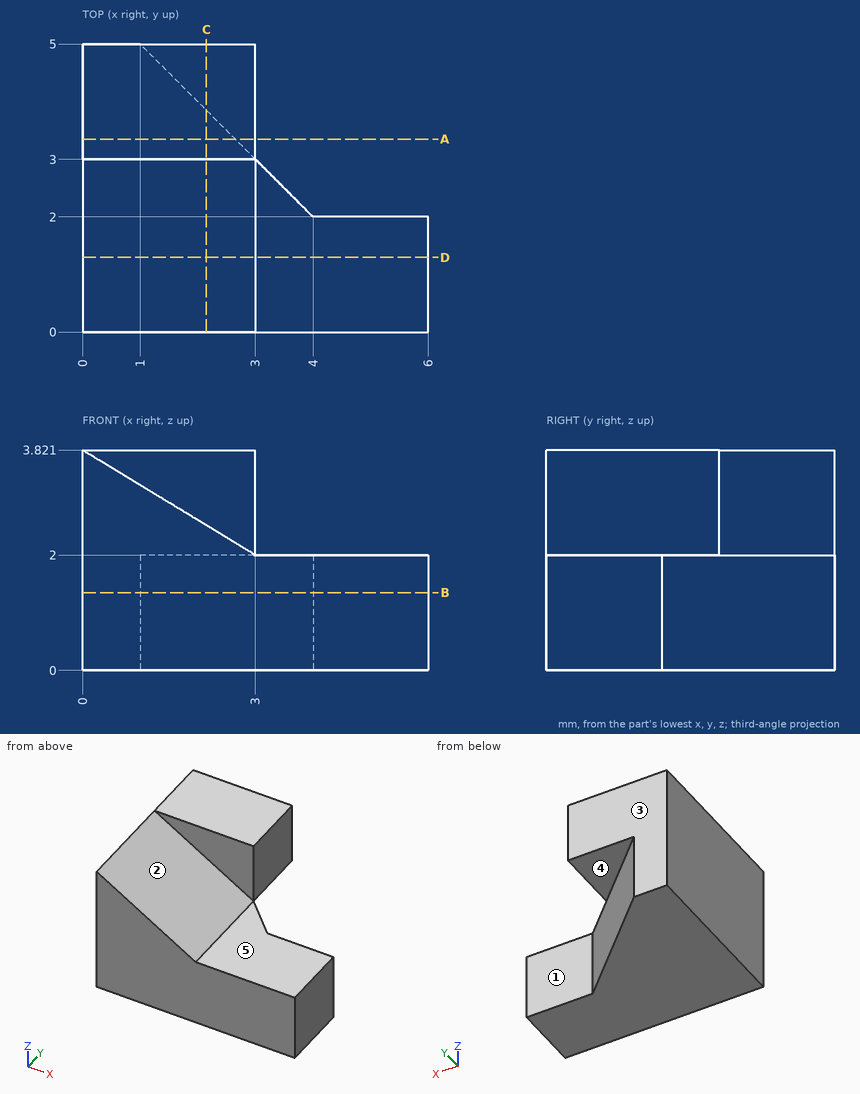
Geometry check sheet. Reference: drawing and pictorial views, mm from the part's lowest x, y, z. A direction names the side the tool comes from. Round coordinates to 2 decimals unless told otherwise and drop trailing zeros. Loops run counter-clockwise (first coordinate to the right, second up) from the corner with the lowest first, then second, coordinate; pieces in that order, holes last. Notation, with made-up numbers: (39.5, 4.5) -> (64.5, 4.5) arc R6 cw to (64.5, 9.5) -> close; hole circle Ø2 at (70.25, -3). An arc over 180 degrees is marked (long way). Use a Markdown table: item, result.
(1) Set-up check for the marked faces 1, 2, 3, 4 and 5: record each of +Z, -Z, +X, -X, +Y, -Y from which the full face is reachable in a straight line by a thin tool's end or side.
Calculated:
| item | result |
|---|---|
| face 1 | +Z, -Z, +X, +Y |
| face 2 | +Z, +X, -Y |
| face 3 | +Z, -Z, +X, -X, +Y |
| face 4 | -Z, +X, +Y |
| face 5 | +Z, +X, +Y, -Y |
(2) Go/stop test with flat-tipped pins: P1, Ø2, axis at y = 4, z = 0.5, coming from the +X side; P2, Ø1.5, axis at x = 5, y = 1.5, coming from the +Z side; P3, Ø2, axis at x = 5, z = 2.5, coming from the +Y side. Record where each tip stops, or that it passes through.
Calculated:
| item | result |
|---|---|
| P1 | x = 3 |
| P2 | z = 2 |
| P3 | y = 2 |
(3) Sectioned sample at B-B (z = 1.35). Enter the section's corners in (x, y).
Calculated:
| item | result |
|---|---|
| outline | (0, 0) -> (6, 0) -> (6, 2) -> (4, 2) -> (1, 5) -> (0, 5) -> close |
(4) Sectioned sample at A-A (y = 3.35). Enter the section's corners in (x, z), then the cut area to 3 significant figures.
Calculated:
| item | result |
|---|---|
| outline | (0, 0) -> (2.65, 0) -> (2.65, 2) -> (3, 2) -> (3, 3.82) -> (0, 3.82) -> close |
| area | 10.8 mm² |
(5) Sectioned sample at D-D (y = 1.3). Enter the section's corners in (x, z).
Calculated:
| item | result |
|---|---|
| outline | (0, 0) -> (6, 0) -> (6, 2) -> (3, 2) -> (0, 3.82) -> close |
(6) Scan lines: probe 1 along Y at (x, z) = (4.6, 1.65); probe 2 along X at (y, z) = (3.05, 3.6). Record each from-to range of solid material in increasing order.
Calculated:
| item | result |
|---|---|
| probe 1 | 0 to 2 |
| probe 2 | 0 to 3 |
(7) Sectioned sample at C-C (x = 2.15). Enter the section's corners in (y, z), then the cut area to 3 significant figures.
Calculated:
| item | result |
|---|---|
| outline | (0, 0) -> (3.85, 0) -> (3.85, 2) -> (5, 2) -> (5, 3.82) -> (3, 3.82) -> (3, 2.52) -> (0, 2.52) -> close |
| area | 12.9 mm² |
